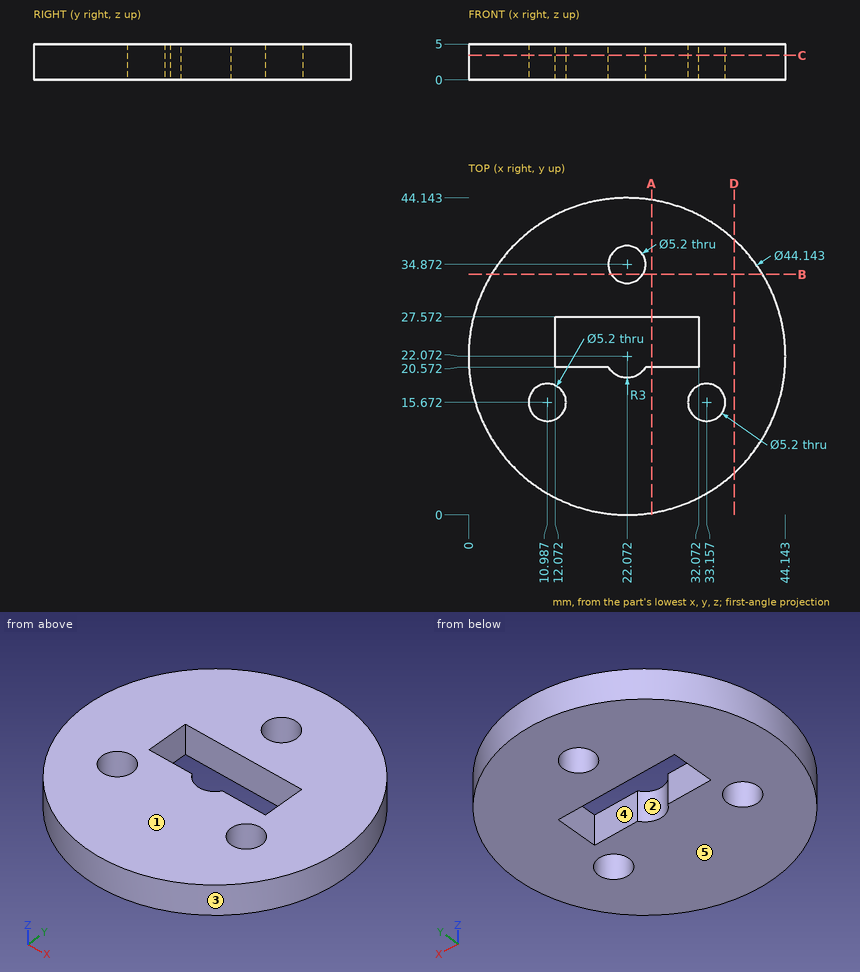
Could you check a few things on this drawing? It's one solid part, dimensions in mm from its lowest x, y, z. A direction names the side the tool comes from. Give positions to 0.01 mm unless a question says otherwise; leave off trailing zeros. Write each loop counter-clockwise with the first axis right and the second up, starting at its lowest first coordinate (ties: lowest second). Pieces come first, ordered by that corner, then holes.
(1) On a 3-axis mill with a long thin cutter (end or side, diameter ignored), from which of +Z, -Z, +X, -X, +Y, -Y can I reach the whole of each face in a straight line? I mean the marked faces 1 and 2. Say none if no direction works.
Output values:
face 1: +Z, +X, -X, +Y, -Y
face 2: +Z, -Z
(2) Will these pins go through, and if not, where does the flat tip stop? pin 1 (1.5 mm diameter, centred on y = 25, z = 3.5, fed in from +X) (1 decimal); pin 2 (2.5 mm diameter, centred on x = 24, z = 3.5, fed in from -Y); pin 3 (1 mm diameter, centred on y = 35.5, z = 3.5, fed in from -X).
Output values:
pin 1: stops at x = 44
pin 2: stops at y = 0.01
pin 3: stops at x = 4.18
(3) Imagine slicing it at C-C, the plane z = 3.4. Write out the boundary of the cut face in (x, y), and give its area (3 significant figures).
Output values:
outline: circle Ø44.14 at (22.07, 22.07); hole circle Ø5.2 at (10.99, 15.67); hole (12.07, 20.57) - (19.47, 20.57) arc R3 ccw to (24.67, 20.57) - (32.07, 20.57) - (32.07, 27.57) - (12.07, 27.57) - close; hole circle Ø5.2 at (22.07, 34.87); hole circle Ø5.2 at (33.16, 15.67)
area: 1,320 mm2
(4) Imagine slicing it at D-D, the plane x = 37. Write out the boundary of the cut face in (y, z) (1 decimal).
Output values:
outline: (5.8, 0) - (38.3, 0) - (38.3, 5) - (5.8, 5) - close
(5) Imagine slicing it at A-A, the plane x = 25.5. Write out the boundary of the cut face in (y, z) (1 decimal).
Output values:
outline: (0.3, 0) - (20.6, 0) - (20.6, 5) - (0.3, 5) - close; (27.6, 0) - (43.9, 0) - (43.9, 5) - (27.6, 5) - close
(6) Thinking about a two-plate mould opening in Y: for the marked faces 3, 4 and 5, which applies, pulls with the +Y half, pulls with the -Y half, needs draft (parallel to the pull), parting line crosses it, or undercut?
Output values:
face 3: parting line crosses it
face 4: undercut
face 5: needs draft
(7) If I drill on L1, parallel to X at y = 13.5, z = 3.75 (1 decimal); L2, parallel to Y at x = 24, z = 1.1 (1 decimal); L3, parallel to X at y = 20, z = 0.55 (1 decimal), over which ranges is the centre line in solid material (lowest first)?
Output values:
L1: x = 1.7 to 9.6, 12.4 to 31.7, 34.6 to 42.4
L2: y = 0.1 to 19.8, 27.6 to 33.1, 36.6 to 44.1
L3: x = 0.1 to 19.9, 24.2 to 44
(8) Imagine slicing it at B-B, the plane y = 33.5. Write out the boundary of the cut face in (x, z) (1 decimal).
Output values:
outline: (3.2, 0) - (19.9, 0) - (19.9, 5) - (3.2, 5) - close; (24.3, 0) - (41, 0) - (41, 5) - (24.3, 5) - close
